from build123d import *

# Parameters (mm, degrees)
ESQUISSE1_R             = 1
ESQUISSE1_R_2           = 0.5
BOSS_EXTRU_1_DEPTH      = 1.5
ESQUISSE3_R             = 3.5
ESQUISSE3_R_2           = 1
BOSS_EXTRU_2_DEPTH      = 2
ESQUISSE4_R             = 2.45
ENL_V_MAT_EXTRU_1_DEPTH = 2


with BuildPart() as part:
    # Esquisse1 → Boss.-Extru.1 (new body)
    with BuildSketch(Plane.XY):
        with BuildLine():
            Line((-1.989974874, 15.2), (-3.48245603, 0.35))
            ThreePointArc((-3.48245603, 0.35), (0, -3.5), (3.48245603, 0.35))
            Line((3.48245603, 0.35), (1.989974874, 15.2))
            ThreePointArc((1.989974874, 15.2), (0, 17), (-1.989974874, 15.2))
        make_face()
        Circle(ESQUISSE1_R, mode=Mode.SUBTRACT)
        with Locations((0, 15)):
            Circle(ESQUISSE1_R_2, mode=Mode.SUBTRACT)
        with Locations((0, 13)):
            Circle(ESQUISSE1_R_2, mode=Mode.SUBTRACT)
        with Locations((0, 11)):
            Circle(ESQUISSE1_R_2, mode=Mode.SUBTRACT)
        with Locations((0, 9)):
            Circle(ESQUISSE1_R_2, mode=Mode.SUBTRACT)
        with Locations((0, 7)):
            Circle(ESQUISSE1_R_2, mode=Mode.SUBTRACT)
        with Locations((0, 5)):
            Circle(ESQUISSE1_R_2, mode=Mode.SUBTRACT)
    extrude(amount=BOSS_EXTRU_1_DEPTH)

    # Esquisse3 → Boss.-Extru.2 (add)
    with BuildSketch(Plane.XY.offset(1.5)):
        Circle(ESQUISSE3_R)
        Circle(ESQUISSE3_R_2, mode=Mode.SUBTRACT)
    extrude(amount=BOSS_EXTRU_2_DEPTH)

    # Esquisse4 → Enlèv. mat.-Extru.1 (cut)
    with BuildSketch(Plane.XY.offset(3.5)):
        Circle(ESQUISSE4_R)
    extrude(amount=-ENL_V_MAT_EXTRU_1_DEPTH, mode=Mode.SUBTRACT)


solid = part.part
Geometry: final body of the model. Coordinates: model frame, mm. A direction names the side the tool comes from. Round coordinates to 2 decimals unless told otherwise and drop trailing zeros. Order: outer loops, then holes, each group sorted by start corner. A loop starts at its lowest first (then second) coordinate and runs counter-clockwise, first axis right, second up.
Q1. Mould query, pull axis X, two halves, no side actions, for faces 1 (the face through (2.747, 7.671, 0.74)), 2 (the face through (2, -2, 3.5)), 3 (the face through (-0.065, 15.496, 0.74)). Classes: released by +X, released by -X, zero draft, split by the parting line, or undercut.
Result sheet:
face 1: released by +X
face 2: zero draft
face 3: undercut
Q2. Section A-A, the plane y = 0. Output: boundary loops of the cut face in (x, z), and give its area (3 significant figures).
Result sheet:
outline: (-3.5, 0) - (-1, 0) - (-1, 1.5) - (-2.45, 1.5) - (-2.45, 3.5) - (-3.5, 3.5) - close; (1, 0) - (3.5, 0) - (3.5, 3.5) - (2.45, 3.5) - (2.45, 1.5) - (1, 1.5) - close
area: 11.7 mm2
Q3. Material intervals for probe 1 along Y at (x, z) = (0, 2.6); probe 2 along Y at (x, z) = (-2.5, 2.9); probe 3 along X at (y, z) = (0, 1.15), sorted ascending.
Result sheet:
probe 1: y = -3.5 to -2.45, 2.45 to 3.5
probe 2: y = -2.45 to 2.45
probe 3: x = -3.5 to -1, 1 to 3.5
Q4. Section D-D, the plane y = 15. Output: boundary loops of the cut face in (x, z), and give its area (3 significant figures).
Result sheet:
outline: (-2.01, 0) - (-0.5, 0) - (-0.5, 1.5) - (-2.01, 1.5) - close; (0.5, 0) - (2.01, 0) - (2.01, 1.5) - (0.5, 1.5) - close
area: 4.53 mm2
Q5. Section B-B, the plane z = 1. Output: boundary loops of the cut face in (x, y), and give its area (3 significant figures).
Result sheet:
outline: (-3.48, 0.35) arc R3.5 ccw (long way) to (3.48, 0.35) - (1.99, 15.2) arc R2 ccw to (-1.99, 15.2) - close; hole circle Ø2 at (0, 0); hole circle Ø1 at (0, 5); hole circle Ø1 at (0, 7); hole circle Ø1 at (0, 9); hole circle Ø1 at (0, 11); hole circle Ø1 at (0, 13); hole circle Ø1 at (0, 15)
area: 101 mm2
Q6. Section C-C, the plane x = 0. Give the number of separate pieces and of enclosed holes in the cut face, and give its area (4 significant figures).
Result sheet:
separate pieces: 8
enclosed holes: 0
area: 22.95 mm2
Q7. Access query for faces 4 (the face through (0.231, 12.556, 0.74)), 5 (the face through (1, -1, 1.5)). Directions: +Z, -Z, +X, -X, +Y, -Y. A direction counts if a zero-diameter tool reaches every point of the face in a straight line with its end or side. Return the directions, or none.
Result sheet:
face 4: +Z, -Z
face 5: +Z
Q8. Pin query (flat end, axial travel): pin 1 (2 mm diameter, centred on x = 0, y = 12, fed in from +Z); pin 2 (2 mm diameter, centred on y = 12, z = 1, fed in from -X); pin 3 (2 mm diameter, centred on y = 2, z = 2, fed in from -X). Return the tip coordinate at first contact, or that it passes through.
Result sheet:
pin 1: stops at z = 1.5
pin 2: stops at x = -2.41
pin 3: stops at x = -3.4
